Work out the finished part from the listing and answer in its coordinate system (mm). Face numbers are marked on the shaded views. Give positions to 0.01 mm unless a question says otherwise; leave off trailing zeros. Order: outer loops, then holes, each group sorted by start corner. A loop starts at its lowest first (then second) coordinate and runs counter-clockwise, first axis right, second up. Notation, with made-up numbers: M -17.75,45.5 L 14.25,45.5 A18 cw 14.25,66.5 Z; hole C 60,28.25 d3. An arc over 180 degrees is marked long. One line per item, written item: value.
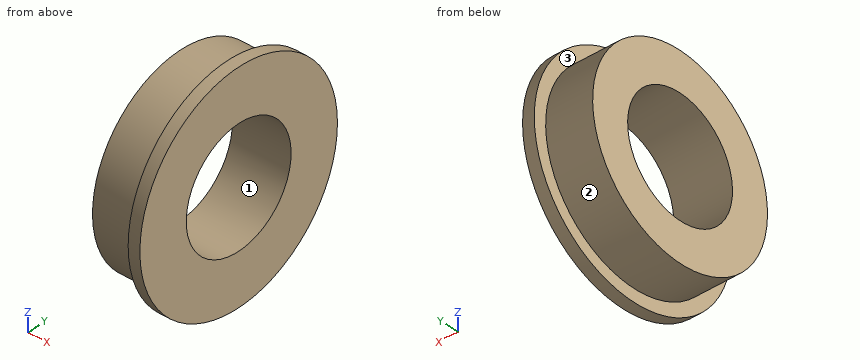
Autodesk Inventor part; units mm, degrees
ref_plane "YZ Plane" through (0, 0, 0) normal (1, 0, 0) x (0, 1, 0)
ref_plane "XZ Plane" through (0, 0, 0) normal (0, 1, 0) x (-1, 0, 0)
ref_plane "XY Plane" through (0, 0, 0) normal (0, 0, 1) x (1, 0, 0)
sketch "スケッチ1" plane through (0, 0, 0) normal (1, 0, 0) x (0, 1, 0)
  circle A0 centre (0, 0) radius 5.65
  dimension "d0" = 11.3
extrude "押し出し1" add sketch "スケッチ1" along normal blind 3
sketch "スケッチ2" plane through (0, 0, 0) normal (-1, 0, 0) x (0, 0, 1)
  circle A0 centre (0, 0) radius 5
  circle A1 centre (0, 0) radius 5.65
  dimension "d3" = 10
extrude "押し出し2" cut sketch "スケッチ2" against normal blind 2.4
sketch "スケッチ3" plane through (0, 0, 0) normal (-1, 0, 0) x (0, 0, 1)
  circle A0 centre (0, 0) radius 3
  dimension "d6" = 6
extrude "押し出し3" cut sketch "スケッチ3" against normal blind 3
properties part number "6mmベアリング"
(1) Given P1, Ø1, axis at x = 2.5, y = -1, coming from the -Z side; P2, Ø1.5, axis at x = 0.5, y = -3.5, coming from the +Z side, each flat-ended and moving along its own axis, determine where each tip first touches the part or whether it passes through.
Findings:
P1: stops at z = -5.63
P2: stops at z = 4.18
(2) Section B-B, the plane z = 0.5 is taken. Give the vertices of the cut face in (x, y), then the cut area to 3 significant figures.
Findings:
outline: M 0,-4.97 L 2.4,-4.97 L 2.4,-5.63 L 3,-5.63 L 3,-2.96 L 0,-2.96 Z; M 0,2.96 L 3,2.96 L 3,5.63 L 2.4,5.63 L 2.4,4.97 L 0,4.97 Z
area: 12.9 mm^2
(3) Find the intervals of material crossed by probe 1 along Y at (x, z) = (1.65, 0); probe 2 along Y at (x, z) = (1.1, -2.25); probe 3 along Z at (x, y) = (2.25, -1.25), in increasing order. Write a range as from..to.
Findings:
probe 1: y = -5..-3, 3..5
probe 2: y = -4.47..-1.98, 1.98..4.47
probe 3: z = -4.84..-2.73, 2.73..4.84
(4) Section D-D, the plane y = -3.5 is taken. Give the vertices of the cut face in (x, z), then the cut area to 3 significant figures.
Findings:
outline: M 0,-3.57 L 2.4,-3.57 L 2.4,-4.44 L 3,-4.44 L 3,4.44 L 2.4,4.44 L 2.4,3.57 L 0,3.57 Z
area: 22.5 mm^2
(5) Section C-C, the plane x = 2.8 is taken. Give the vertices of the cut face in (y, z), then the cut area to 3 significant figures.
Findings:
outline: C 0,0 d11.3; hole C 0,0 d6
area: 72.0 mm^2
(6) Section A-A, the plane y = 0 is taken. Give the vertices of the cut face in (x, z), then the cut area to 3 significant figures.
Findings:
outline: M 0,-5 L 2.4,-5 L 2.4,-5.65 L 3,-5.65 L 3,-3 L 0,-3 Z; M 0,3 L 3,3 L 3,5.65 L 2.4,5.65 L 2.4,5 L 0,5 Z
area: 12.8 mm^2
(7) Determine the mould class of the marked faces 1, 2 and 3 for opening direction Z: pulls with the +Z half, pulls with the -Z half, needs draft (parallel to the pull), parting line crosses it, or undercut.
Findings:
face 1: undercut
face 2: parting line crosses it
face 3: needs draft
